Verification items for this drawing (mm, ordinates from the low corner). A direction names the side the tool comes from. Round coordinates to 2 decimals unless told otherwise and drop trailing zeros. Loops run counter-clockwise (first coordinate to the right, second up) from the corner with the lowest first, then second, coordinate; pieces in that order, holes last. Notation, with made-up numbers: M 46,41.25 L 103,41.25 A19 cw 103,47.25 Z; hole C 70,36 d8. An arc over 180 degrees is marked long. Answer in a Markdown table with one row per item. Add a question column.
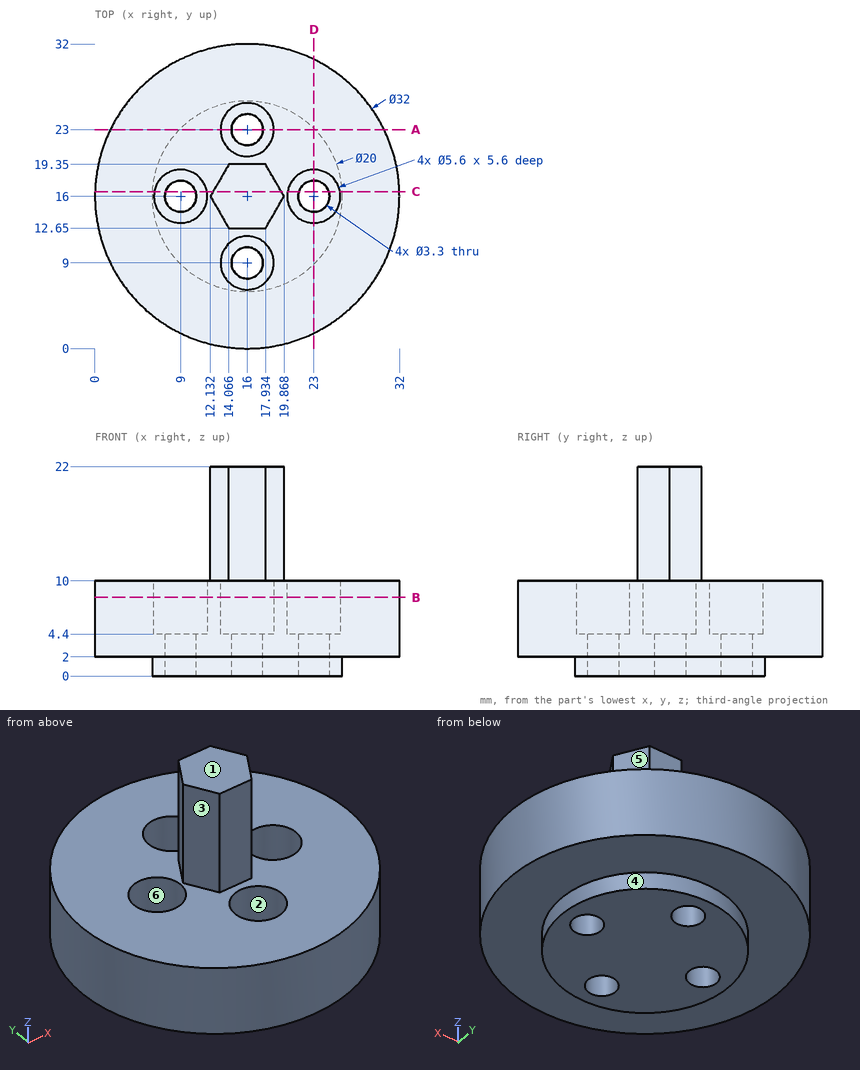
1) Thickness scan on L1, parallel to Y at x = 16, z = 6.55; L2, parallel to Y at x = 16, z = 1.95; L3, parallel to Z at x = 29.5, y = 7.5. Record the ranges inside material, lowest first. Write a range as [from, to].
2) Draft check along Y on the marked faces 1, 2 and 3. Enter one of: +Y half, -Y half, draft (parallel to the pull), parting line (faces both ways), or undercut.
3) Go/stop test with flat-tipped pins: pin 1 (4.5 mm diameter, centred on x = 17, y = 9, fed in from +Z); pin 2 (3 mm diameter, centred on x = 14, z = 13, fed in from +Y); pin 3 (12 mm diameter, centred on y = 21, z = 19.5, fed in from +X); pin 4 (2 mm diameter, centred on x = 3.5, z = 12.5, fed in from -Y). Record where each tip stops, or that it passes through.
4) Set-up check for the marked faces 4, 5 and 6: record each of +Z, -Z, +X, -X, +Y, -Y from which the full face is reachable in a straight line by a thin tool's end or side.
5) Cross-section at C-C, the plane y = 16.5. Record the boundary of the cut face in (x, z) (1 decimal), plus the area to 3 significant figures.
6) Cross-section at A-A, the plane y = 23. Record the boundary of the cut face in (x, z).
7) Cross-section at B-B, the plane z = 8.25. Record the boundary of the cut face in (x, y), plus the area to 3 significant figures.
Worked answers:
| question | item | result |
|---|---|---|
| 1 | L1 | y = [0, 6.2], [11.8, 20.2], [25.8, 32] |
| 1 | L2 | y = [6, 7.35], [10.65, 21.35], [24.65, 26] |
| 1 | L3 | z = [2, 10] |
| 2 | face 1 | draft |
| 2 | face 2 | undercut |
| 2 | face 3 | -Y half |
| 3 | pin 1 | stops at z = 10 |
| 3 | pin 2 | stops at y = 19.35 |
| 3 | pin 3 | stops at x = 19.87 |
| 3 | pin 4 | passes through |
| 4 | face 4 | -Z |
| 4 | face 5 | +Z, +X, +Y |
| 4 | face 6 | +Z |
| 5 | outline | M 0,2 L 6,2 L 6,0 L 7.4,0 L 7.4,4.4 L 6.2,4.4 L 6.2,10 L 0,10 Z; M 10.6,0 L 21.4,0 L 21.4,4.4 L 20.2,4.4 L 20.2,10 L 19.6,10 L 19.6,22 L 12.4,22 L 12.4,10 L 11.8,10 L 11.8,4.4 L 10.6,4.4 Z; M 24.6,0 L 26,0 L 26,2 L 32,2 L 32,10 L 25.8,10 L 25.8,4.4 L 24.6,4.4 Z |
| 5 | area | 292 mm2 |
| 6 | outline | M 1.61,2 L 8.86,2 L 8.86,0 L 14.35,0 L 14.35,4.4 L 13.2,4.4 L 13.2,10 L 1.61,10 Z; M 17.65,0 L 23.14,0 L 23.14,2 L 30.39,2 L 30.39,10 L 18.8,10 L 18.8,4.4 L 17.65,4.4 Z |
| 7 | outline | C 16,16 d32; hole C 9,16 d5.6; hole C 16,9 d5.6; hole C 16,23 d5.6; hole C 23,16 d5.6 |
| 7 | area | 706 mm2 |
